```python
from build123d import *

# Parameters (mm, degrees)
SKETCH1_W               = 50
SKETCH1_H               = 50
SKETCH1_R               = 3.5
BOSS_EXTRUDE1_DEPTH     = 4
SKETCH2_W               = 25
SKETCH2_H               = 25
SKETCH2_W_2             = 19
SKETCH2_H_2             = 19
BOSS_EXTRUDE2_DEPTH     = 22.5
CUT_EXTRUDE1_DEPTH      = 53.282884389
CUT_EXTRUDE1_DEPTH_BACK = 53.282884389
SKETCH3_R               = 2.75
CUT_EXTRUDE2_DEPTH      = 53.282884389
CUT_EXTRUDE2_DEPTH_BACK = 53.282884389
SKETCH4_R               = 2.75


with BuildPart() as part:
    # Sketch1 → Boss-Extrude1 (new body)
    with BuildSketch(Plane(origin=(0, 0, 0), x_dir=(1, 0, 0), z_dir=(0, 1, 0))):
        Rectangle(SKETCH1_W, SKETCH1_H)
        with Locations(Location((-17.5, -17.5, 0), (0, 0, 270))):
            Circle(SKETCH1_R, mode=Mode.SUBTRACT)
        with Locations(Location((17.5, -17.5, 0), (0, 0, 270))):
            Circle(SKETCH1_R, mode=Mode.SUBTRACT)
        with Locations(Location((17.5, 17.5, 0), (0, 0, 270))):
            Circle(SKETCH1_R, mode=Mode.SUBTRACT)
        with Locations(Location((-17.5, 17.5, 0), (0, 0, 270))):
            Circle(SKETCH1_R, mode=Mode.SUBTRACT)
    extrude(amount=BOSS_EXTRUDE1_DEPTH)

    # Sketch2 → Boss-Extrude2 (add)
    with BuildSketch(Plane(origin=(0, 4, 0), x_dir=(1, 0, 0), z_dir=(0, 1, 0))):
        Rectangle(SKETCH2_W, SKETCH2_H)
        Rectangle(SKETCH2_W_2, SKETCH2_H_2, mode=Mode.SUBTRACT)
    extrude(amount=BOSS_EXTRUDE2_DEPTH)

    # Sketch3 → Cut-Extrude1 (cut, two sides: drawn at the far end of the back side and taken through both)
    with BuildSketch(Plane.ZY.offset(12.5).offset(-CUT_EXTRUDE1_DEPTH_BACK)):
        with Locations((0, 20.5)):
            Circle(SKETCH3_R)
    extrude(amount=CUT_EXTRUDE1_DEPTH + CUT_EXTRUDE1_DEPTH_BACK, mode=Mode.SUBTRACT)

    # Sketch4 → Cut-Extrude2 (cut, two sides: drawn at the far end of the back side and taken through both)
    with BuildSketch(Plane.XY.offset(12.5).offset(-CUT_EXTRUDE2_DEPTH_BACK)):
        with Locations((0, 20.5)):
            Circle(SKETCH4_R)
    extrude(amount=CUT_EXTRUDE2_DEPTH + CUT_EXTRUDE2_DEPTH_BACK, mode=Mode.SUBTRACT)


solid = part.part
```
Input: part model. Units: mm. Frame: model coordinates. A direction names the side the tool comes from. Round coordinates to 2 decimals unless told otherwise and drop trailing zeros. Loops run counter-clockwise (first coordinate to the right, second up) from the corner with the lowest first, then second, coordinate; pieces in that order, holes last. Notation, with made-up numbers: M -9.75,61.25 L 20.25,61.25 A27 ccw 20.25,84.25 Z; hole C 45.5,73.5 d6. An arc over 180 degrees is marked long. Answer in a Markdown table with one row per item. Add a question column.
1. Mould query, pull axis Y, two halves, no side actions, for faces 4 (the face through (-0.358, 23.227, 10.979)), 5 (the face through (11.021, 23.227, -0.358)), 6 (the face through (-12.5, 15, 0)), 7 (the face through (-11, 26.5, 0)). Classes: released by +Y, released by -Y, zero draft, split by the parting line, or undercut.
2. Section A-A (y = 16.5). Output: boundary loops of the cut face in (x, z), and give its area (3 significant figures).
3. Contact query for flat-ended pins moving along their axis: pin 1 (15 mm diameter, centred on x = -0.5, y = 15.5, fed in from -Z); pin 2 (4 mm diameter, centred on x = -4, y = 15.5, fed in from +Z); pin 3 (5.5 mm diameter, centred on y = 9.5, z = -3.5, fed in from -X); pin 4 (21 mm diameter, centred on x = 3, z = 1.5, fed in from +Y). Output: stop coordinate, or through.
4. Section C-C (x = 17.5). Output: boundary loops of the cut face in (y, z), and give its area (3 significant figures).
5. Set-up query: faces 1 (the face through (0, 15, -12.5)), 2 (the face through (0, 15, 12.5)), 3 (the face through (0, 15, -9.5)). Return all of +Z, -Z, +X, -X, +Y, -Y with unobstructed straight access to the full face (end or side cutting, diameter ignored); none if empty.
6. Section B-B (z = 10.5). Output: boundary loops of the cut face in (x, y), and give its area (3 significant figures).
7. Ray query, probe 1 along X at (y, z) = (1.2, -17.5); probe 2 along Y at (x, z) = (0, -10); probe 3 along X at (y, z) = (24, -3). Return the intervals inside material, ascending.
8. Section D-D (y = 2). Output: boundary loops of the cut face in (x, z), and give its area (3 significant figures).
Values follow:
| question | item | result |
|---|---|---|
| 1 | face 4 | undercut |
| 1 | face 5 | undercut |
| 1 | face 6 | zero draft |
| 1 | face 7 | released by +Y |
| 2 | outline | M -12.5,-12.5 L 12.5,-12.5 L 12.5,12.5 L -12.5,12.5 Z; hole M -9.5,-9.5 L 9.5,-9.5 L 9.5,9.5 L -9.5,9.5 Z |
| 2 | area | 264 mm^2 |
| 3 | pin 1 | z = -12.5 |
| 3 | pin 2 | z = 12.5 |
| 3 | pin 3 | x = -12.5 |
| 3 | pin 4 | y = 26.5 |
| 4 | outline | M 0,-25 L 4,-25 L 4,-21 L 0,-21 Z; M 0,-14 L 4,-14 L 4,14 L 0,14 Z; M 0,21 L 4,21 L 4,25 L 0,25 Z |
| 4 | area | 144 mm^2 |
| 5 | face 1 | -Z, +X, -X, +Y |
| 5 | face 2 | +Z, +X, -X, +Y |
| 5 | face 3 | +Y |
| 6 | outline | M -25,0 L 25,0 L 25,4 L 12.5,4 L 12.5,26.5 L -12.5,26.5 L -12.5,4 L -25,4 Z; hole C 0,20.5 d5.5 |
| 6 | area | 739 mm^2 |
| 7 | probe 1 | -25 to -21, -14 to 14, 21 to 25 |
| 7 | probe 2 | 0 to 17.75, 23.25 to 26.5 |
| 7 | probe 3 | -12.5 to -9.5, 9.5 to 12.5 |
| 8 | outline | M -25,-25 L 25,-25 L 25,25 L -25,25 Z; hole C -17.5,-17.5 d7; hole C -17.5,17.5 d7; hole C 17.5,-17.5 d7; hole C 17.5,17.5 d7 |
| 8 | area | 2,350 mm^2 |
